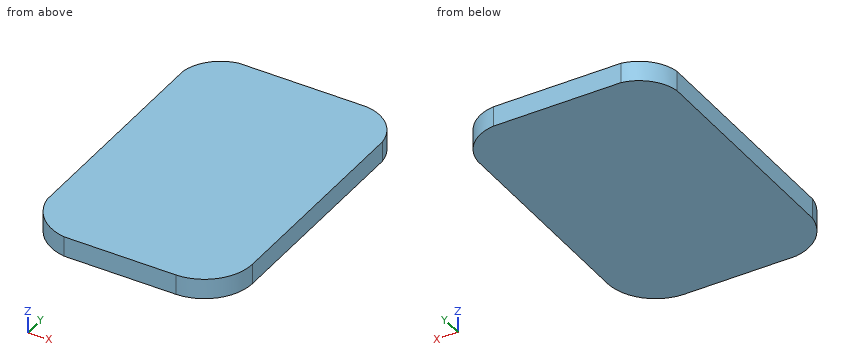
from build123d import *

# Parameters (mm, degrees)
BOSS_EXTRUDE1_DEPTH = 120


with BuildPart() as part:
    # Sketch3 → Boss-Extrude1 (new body)
    with BuildSketch(Plane.XY):
        with BuildLine():
            Line((367.047667182, 900), (-392.766729868, 900))
            ThreePointArc((-392.766729868, 900), (-529.765209749, 829.765209749), (-600, 692.766729868))
            Line((-600, 692.766729868), (-600, -652.262218358))
            ThreePointArc((-600, -652.262218358), (-516.83040869, -816.83040869), (-352.262218358, -900))
            Line((-352.262218358, -900), (316.675693069, -900))
            ThreePointArc((316.675693069, -900), (515.76634783, -815.76634783), (600, -616.675693069))
            Line((600, -616.675693069), (600, -607.982402727))
            Line((600, -607.982402727), (600, 671.022296826))
            ThreePointArc((600, 671.022296826), (524.004104789, 826.694082288), (367.047667182, 900))
        make_face()
    extrude(amount=BOSS_EXTRUDE1_DEPTH)


solid = part.part
Input: part model. Units: mm. Frame: model coordinates. Give positions to 0.01 mm unless a question says otherwise; leave off trailing zeros. Order: outer loops, then holes, each group sorted by start corner. A loop starts at its lowest first (then second) coordinate and runs counter-clockwise, first axis right, second up. Notation, with made-up numbers: (4.25, 70) - (8.25, 70) arc R20 ccw to (8.25, 76) - close; hole circle Ø2 at (-2, 72). An arc over 180 degrees is marked (long way). Answer as a JSON object with one key per item and string values. Group by question number.
Q1. Cut plane C-C, the plane x = 504. Output: boundary loops of the cut face in (y, z).
Q2. Line query: probe 1 along Y at (x, z) = (-412, 69.5); probe 2 along Y at (x, z) = (525.5, 41); probe 3 along X at (y, z) = (799.5, 16.5). Output: solid intervals per line, ascending.
Q3. Cut plane A-A, the plane z = 68.5. Output: boundary loops of the cut face in (x, y), then the cut area to 3 significant figures.
Q4. First-contact query: pin 1 Ø2 at (x, y) = (-103, 465) entering from -Z. Flat tip, straight axial feed; report the tip coordinate or a pass-through.
Q5. Cut plane B-B, the plane y = 725. Output: boundary loops of the cut face in (x, z).
Results:
{
 "1": {"outline": "(-826.89, 0) - (844.43, 0) - (844.43, 120) - (-826.89, 120) - close"},
 "2": {"probe 1": "-884.42 to 896.08", "probe 2": "-805.54 to 825.21", "probe 3": "-555.57 to 548.05"},
 "3": {"outline": "(-600, -652.26) arc R295.36 ccw to (-352.26, -900) - (316.68, -900) arc R287.7 ccw to (600, -616.68) - (600, 671.02) arc R259.83 ccw to (367.05, 900) - (-392.77, 900) arc R251.03 ccw to (-600, 692.77) - close", "area": "2,100,000 mm^2"},
 "4": {"pin 1": "z = 0"},
 "5": {"outline": "(-592.52, 0) - (587.88, 0) - (587.88, 120) - (-592.52, 120) - close"}
}
